Check sheet for the modelled part. Datum: model origin and axes. Units: mm. Face numbers are marked on the shaded views. A direction names the side the tool comes from. Round coordinates to 2 decimals unless told otherwise and drop trailing zeros. Loops run counter-clockwise (first coordinate to the right, second up) from the corner with the lowest first, then second, coordinate; pieces in that order, holes last. Notation, with made-up numbers: (-21, 79.5) - (-15, 79.5) arc R25 cw to (-15, 110.5) - close; hole circle Ø1 at (61.25, 60). An arc over 180 degrees is marked (long way). Answer in a Markdown table with one row per item. Add a question column.
(1) Thickness scan on line 1 along Y through (x, z) = (0, 12.75); line 2 along X through (y, z) = (-1.5, 10.15); line 3 along X through (y, z) = (-3, 10.15). Record the ranges inside material, lowest first.
(2) Mould release check, pull along X, two halves, no side actions. Record for the marked faces 1, 2 and 3: +X half, -X half, draft (parallel to the pull), parting line (faces both ways), or undercut.
(3) Cross-section at A-A on y = 0. Enter the section's corners in (x, z), then the cut area to 3 significant figures.
(4) Cross-section at D-D on y = 13. Enter the section's corners in (x, z).
(5) Cross-section at B-B on x = 15. Enter the section's corners in (y, z), then the cut area to 3 significant figures.
(6) Access from +Z, -Z, +X, -X, +Y, -Y to the whole of each face (thin tool, end or side, straight path). Record for the marked faces 4, 5, 6 and 7.
(7) Gauge pin test, flat ends, axial feed: pin 1 (8 mm diameter, centred on x = -13.5, y = -5.5, fed in from -Z); pin 2 (2 mm diameter, centred on x = 5.5, y = -2, fed in from +Z); pin 3 (8 mm diameter, centred on x = 6.5, z = 10.5, fed in from -Y); pin 4 (3 mm diameter, centred on x = 17, z = 6, fed in from -Y). Record the tip position at first contact, or that the pin passes through.
(8) Cross-section at C-C on z = 13.25. Enter the section's corners in (x, y), then the cut area to 3 significant figures.
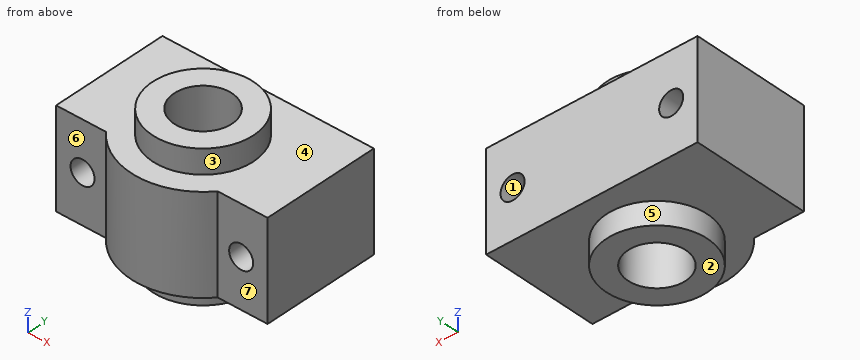
from build123d import *

# Parameters (mm, degrees)
IZIM1_R                          = 6
Y_KSEKLIK_EKSTR_ZYON1_DEPTH      = 20.3
Y_KSEKLIK_EKSTR_ZYON2_DEPTH      = 5
Y_KSEKLIK_EKSTR_ZYON2_DEPTH_BACK = 25
IZIM2_R                          = 10.5
IZIM2_R_2                        = 6
IZIM5_R                          = 2.5
KES_EKSTR_ZYON1_DEPTH            = 45.989887753


with BuildPart() as part:
    # Çizim1 → Yükseklik-Ekstrüzyon1 (new body)
    with BuildSketch(Plane.XY):
        with BuildLine():
            Line((-22, -9.5), (-11.608186766, -9.5))
            ThreePointArc((-11.608186766, -9.5), (0, -15), (11.608186766, -9.5))
            Line((11.608186766, -9.5), (22, -9.5))
            Line((22, -9.5), (22, 15))
            Line((22, 15), (-22, 15))
            Line((-22, 15), (-22, -9.5))
        make_face()
        Circle(IZIM1_R, mode=Mode.SUBTRACT)
    extrude(amount=Y_KSEKLIK_EKSTR_ZYON1_DEPTH)

    # Çizim2 → Yükseklik-Ekstrüzyon2 (add, two sides: drawn at the far end of the back side and taken through both)
    with BuildSketch(Plane.XY.offset(20.3).offset(-Y_KSEKLIK_EKSTR_ZYON2_DEPTH_BACK)):
        Circle(IZIM2_R)
        Circle(IZIM2_R_2, mode=Mode.SUBTRACT)
    extrude(amount=Y_KSEKLIK_EKSTR_ZYON2_DEPTH + Y_KSEKLIK_EKSTR_ZYON2_DEPTH_BACK)

    # Çizim5 → Kes-Ekstrüzyon1 (cut, through all)
    with BuildSketch(Plane(origin=(0, 15, 0), x_dir=(1, 0, 0), z_dir=(0, 1, 0))):
        with Locations(Location((-16.5, -10.15, 0), (0, 0, 270))):
            Circle(IZIM5_R)
        with Locations(Location((16.5, -10.15, 0), (0, 0, 270))):
            Circle(IZIM5_R)
    extrude(amount=-KES_EKSTR_ZYON1_DEPTH, mode=Mode.SUBTRACT)


solid = part.part
Answers:
| question | item | result |
|---|---|---|
| 1 | line 1 | y = -15 to -6, 6 to 15 |
| 1 | line 2 | x = -22 to -19, -14 to -5.81, 5.81 to 14, 19 to 22 |
| 1 | line 3 | x = -22 to -19, -14 to -5.2, 5.2 to 14, 19 to 22 |
| 2 | face 1 | undercut |
| 2 | face 2 | draft |
| 2 | face 3 | parting line |
| 3 | outline | (-22, 0) - (-10.5, 0) - (-10.5, -4.7) - (-6, -4.7) - (-6, 25.3) - (-10.5, 25.3) - (-10.5, 20.3) - (-22, 20.3) - close; (6, -4.7) - (10.5, -4.7) - (10.5, 0) - (22, 0) - (22, 20.3) - (10.5, 20.3) - (10.5, 25.3) - (6, 25.3) - close; hole circle Ø5 at (-16.5, 10.15); hole circle Ø5 at (16.5, 10.15) |
| 3 | area | 698 mm^2 |
| 4 | outline | (-22, 0) - (22, 0) - (22, 20.3) - (-22, 20.3) - close; hole circle Ø5 at (-16.5, 10.15); hole circle Ø5 at (16.5, 10.15) |
| 5 | outline | (-9.5, 0) - (15, 0) - (15, 8.15) - (-9.5, 8.15) - close; (-9.5, 12.15) - (15, 12.15) - (15, 20.3) - (-9.5, 20.3) - close |
| 5 | area | 399 mm^2 |
| 6 | face 4 | +Z |
| 6 | face 5 | -Z |
| 6 | face 6 | +Z, -Z, -X, -Y |
| 6 | face 7 | +Z, -Z, +X, -Y |
| 7 | pin 1 | stops at z = 0 |
| 7 | pin 2 | stops at z = 25.3 |
| 7 | pin 3 | stops at y = -14.79 |
| 7 | pin 4 | stops at y = -9.5 |
| 8 | outline | (-22, -9.5) - (-11.61, -9.5) arc R15 ccw to (11.61, -9.5) - (22, -9.5) - (22, 15) - (-22, 15) - close; hole circle Ø12 at (0, 0) |
| 8 | area | 1,050 mm^2 |
